Autodesk Inventor part; units mm, degrees
ref_plane "XZ Plane" through (0, 0, 0) normal (0, 1, 0) x (-1, 0, 0)
ref_plane "XY Plane" through (0, 0, 0) normal (0, 0, 1) x (1, 0, 0)
sketch "Sketch1" plane through (0, 0, 0) normal (0, 1, 0) x (-1, 0, 0)
  circle A0 centre (0, 0) radius 36
  dimension "d0" = 72
extrude "Extrusion1" add sketch "Sketch1" along normal blind 1.5
sketch "Sketch2" plane through (0, 1.5, 0) normal (0, 1, 0) x (1, 0, 0)
  circle A0 centre (0, 0) radius 36
  circle A1 centre (0, 0) radius 33
  circle A2 centre (0, 0) radius 31
  dimension "d3" = 3
  dimension "d4" = 2
  dimension "d23" = 72
  dimension "d24" = 66
  dimension "d25" = 62
extrude "Extrusion2" add sketch "Sketch2" along normal blind 30 contours A1
sketch "Sketch3" plane through (0, 1.5, 0) normal (0, 1, 0) x (1, 0, 0)
  circle A0 centre (0, 0) radius 36
  circle A1 centre (0, 0) radius 33
  dimension "d51" = 72
  dimension "d52" = 66
extrude "Extrusion3" add sketch "Sketch3" along normal blind 28
sketch "Sketch5" plane through (0, 31.5, 0) normal (0, 1, 0) x (1, 0, 0)
  circle A0 centre (0, 0) radius 22.5
  line L0 (-22.5, 0) -> (7.2195, 0) construction
  line L1 (0, -22.5) -> (23.761, -22.5) construction
  line L2 (22.5, 0) -> (0, -22.5)
  line L3 (0, -22.5) -> (19.2037, -41.7037)
  line L4 (0, -22.5) -> (27.1581, -22.5) construction
  line L5 (22.5, 0) -> (46.5776, -24.0776)
  line L6 (22.5, 0) -> (56.5508, 0) construction
  line L7 (46.5776, -24.0776) -> (19.2037, -41.7037)
  dimension "d13" = 45
  dimension "d18" = 45
  dimension "d19" = 45
extrude "Extrusion4" cut sketch "Sketch5" against normal blind 7 contours L5 L7 L3 A0 | A0 L2 picked at (12.1762, -13.3637)
ref_plane "Work Plane1" through (-36, 0, 0) normal (1, 0, 0) x (0, 1, 0)
sketch "Sketch7" plane through (-36, 0, 0) normal (1, 0, 0) x (0, 1, 0)
  circle A0 centre (24.5, 0) radius 1.5
  line L0 (29.5, -36) -> (29.5, 36)
  point P0 (0, 0)
  point P1 (29.5, 11.585)
  point P2 (29.5, 34.085)
  dimension "d26" = 3
  dimension "d27" = 5
hole "Hole1" at (-36, 24.5, 0) direction (1, 0, 0) diameter 3 depth 8 tip angle 118
ref_plane "Work Plane2" through (36, 0, 0) normal (1, 0, 0) x (0, 1, 0)
sketch "Sketch8" plane through (36, 0, 0) normal (1, 0, 0) x (0, 1, 0)
  circle A0 centre (24.5, 0) radius 1.5
  line L0 (29.5, -36) -> (29.5, 36)
  point P0 (0, 0)
  point P1 (29.5, 11.585)
  point P2 (29.5, 34.085)
  dimension "d42" = 3
  dimension "d43" = 5
hole "Hole2" at (36, 24.5, 0) direction (-1, 0, 0) diameter 3 depth 8 tip angle 118
sketch "Sketch10" plane through (0, 1.5, 0) normal (0, 1, 0) x (1, 0, 0)
  line L0 (0, 0) -> (0, -50)
  line L1 (0, 0) -> (49.9372, -49.9372)
  line L2 (0, 0) -> (70.6219, 0) construction
  line L3 (0, 0) -> (-49.9372, -49.9372)
  line L4 (0, 0) -> (70.6219, 0) construction
  circle A0 centre (0, 0) radius 36
  line L5 (-49.9372, -49.9372) -> (49.9372, -49.9372)
  point P0 (-25.4558, -25.4558)
  point P1 (25.4558, -25.4558)
  dimension "d44" = 50
  dimension "d45" = 45
  dimension "d46" = 135
extrude "Extrusion5" add sketch "Sketch10" along normal blind 21.5 and the other way blind 1.5 contours A0 L1 L5 L0 | L0 L5 L3 A0
properties part number "clock_case_bottom"
Read the model definition and answer for the solid it produces. Units are mm, in the model's axes. A direction names the side the tool comes from. Give positions to 0.01 mm unless a question says otherwise; leave off trailing zeros. Write each loop counter-clockwise with the first axis right and the second up, starting at its lowest first coordinate (ties: lowest second). Pieces come first, ordered by that corner, then holes. Notation, with made-up numbers: (48.25, 3) - (91.25, 3) arc R29 cw to (91.25, 30) - close; hole circle Ø7 at (15, -30). An arc over 180 degrees is marked (long way). Write item = value, one per line. Start each with the question number.
Item 1: The mould has two halves that part along Z. Classify faces 1 (the flat face through (-1, 11, 49.937)), 2 (the flat face through (38, 11, 38)), 3 (the flat face through (-1, 0, 6)): +Z half, -Z half, draft (parallel to the pull), parting line (faces both ways), or undercut.
Item 2: A tool of negligible diameter and unlimited length cuts with its end or side. For faces 4 (the cylindrical face through (33, 23, 0)), 5 (the flat face through (32, 27.3, 9.5)), 6 (the flat face through (9.5, 27.3, 32)), 7 (the flat face through (-38, 11, 38)), 8 (the cylindrical face through (-24.601, 16.29, -18.863)), from which of +Z, -Z, +X, -X, +Y, -Y can it reach the whole face along a straight path? Write none if from no direction.
Item 3: Each of these flat-tipped pins is pushed along its axis until it touches: P1, Ø8, axis at y = 9.5, z = 15, coming from the -X side; P2, Ø2, axis at x = -14.5, y = 15, coming from the -Z side; P3, Ø1.5, axis at y = 21, z = 36, coming from the -X side. Where does it stop, or does it pass through?
Item 4: Find section A-A (z = 0). Give the vertices of the cut face in (x, y), then the cut area to 3 significant figures.
Item 5: Find the intervals of material crossed by probe 1 along Z at (x, y) = (0, 16); probe 2 along Y at (x, z) = (-34, 0); probe 3 along Y at (x, z) = (28, -10), in increasing order. Write a range as [from, to].
Item 6: Find section D-D (x = -34.5). Give the vertices of the cut face in (y, z), then the cut area to 3 significant figures.
Item 7: Find section C-C (y = 18.5). Give the vertices of the cut face in (x, z).
Item 8: Find section B-B (x = 0). Give the vertices of the cut face in (y, z).
Response:
q1.face_1 = +Z half
q1.face_2 = undercut
q1.face_3 = draft
q2.face_4 = +X, -X
q2.face_5 = +Z, +Y
q2.face_6 = +X, +Y
q2.face_7 = -X, +Y, -Y
q2.face_8 = +Y
q3.P1 = -34.28
q3.P2 = -33.37
q3.P3 = -36.75
q4.outline = (-36, 0) - (36, 0) - (36, 23) - (31, 23) - (31, 1.5) - (-31, 1.5) - (-31, 23) - (-36, 23) - close; (-36, 26) - (-31, 26) - (-31, 31.5) - (-33, 31.5) - (-33, 29.5) - (-36, 29.5) - close; (31, 26) - (36, 26) - (36, 29.5) - (33, 29.5) - (33, 31.5) - (31, 31.5) - close
q4.area = 366 mm²
q5.probe_1 = [-36, -31], [31, 49.94]
q5.probe_2 = [0, 23], [26, 29.5]
q5.probe_3 = [0, 1.5]
q6.outline = (0, -10.28) - (29.5, -10.28) - (29.5, 10.28) - (0, 10.28) - close; (0, 34.5) - (23, 34.5) - (23, 49.94) - (0, 49.94) - close; hole circle Ø3 at (24.5, 0)
q6.area = 955 mm²
q7.outline = (-49.94, 49.94) - (-25.46, 25.46) arc R36 ccw (long way) to (25.46, 25.46) - (49.94, 49.94) - close; hole circle Ø62 at (0, 0)
q8.outline = (0, -36) - (29.5, -36) - (29.5, -33) - (31.5, -33) - (31.5, -31) - (1.5, -31) - (1.5, 31) - (31.5, 31) - (31.5, 33) - (29.5, 33) - (29.5, 36) - (23, 36) - (23, 49.94) - (0, 49.94) - close
